Input: dimensioned drawing with shaded views. Units: mm. Origin: part minimum x, y, z. A direction names the side the tool comes from. Round coordinates to 2 decimals unless told otherwise and drop trailing zeros. Loops run counter-clockwise (first coordinate to the right, second up) from the corner with the lowest first, then second, coordinate; pieces in that order, holes last.
Item 1: Ray query, L1, parallel to X at y = 1.5, z = 6; L2, parallel to X at y = 0.8, z = 11; L3, parallel to X at y = 0.25, z = 13.25. Return the intervals inside material, ascending.
Item 2: First-contact query: P1, Ø0.8, axis at y = 0.5, z = 7, coming from the +X side; P2, Ø1.1, axis at y = 0.5, z = 8.5, coming from the -X side. Flat tips, straight axial feed; report the tip coordinate or a pass-through.
Item 3: Section query B-B on z = 10.5. Return loops of the section in (x, y), then the cut area to 3 significant figures.
Item 4: Pull-direction query (X, two-part tool) for the marked faces 1 and 2; classes: released by +X, released by -X, zero draft, split by the parting line, or undercut.
Item 5: Section query A-A on y = 0.6. Return loops of the section in (x, z).
Item 6: Section query C-C on x = 23.5. Return loops of the section in (y, z).
Item 7: Section query D-D on z = 12.25. Return loops of the section in (x, y), then the cut area to 3 significant figures.
Item 8: Access query for the marked faces 3 and 4. Directions: +Z, -Z, +X, -X, +Y, -Y. A direction counts if a zero-diameter tool reaches every point of the face in a straight line with its end or side. Return the directions, or none.
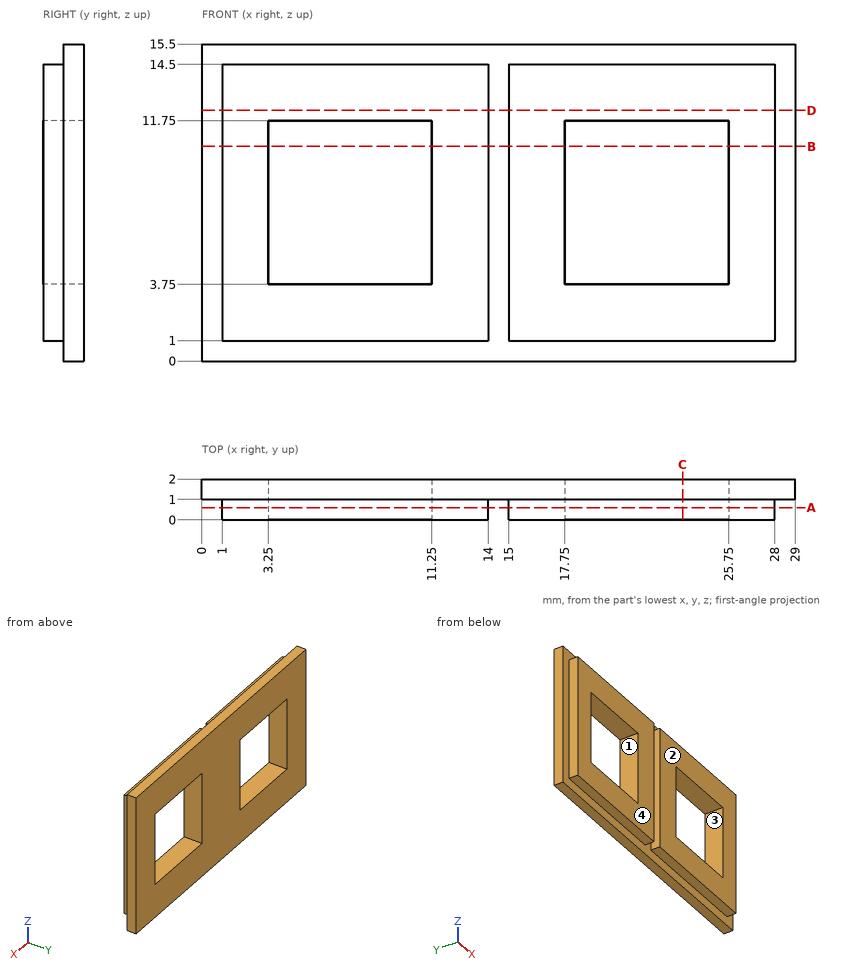
Data:
1. L1: x = 0 to 3.25, 11.25 to 17.75, 25.75 to 29
1. L2: x = 1 to 3.25, 11.25 to 14, 15 to 17.75, 25.75 to 28
1. L3: x = 1 to 14, 15 to 28
2. P1: stops at x = 28
2. P2: stops at x = 0
3. outline: (0, 1) - (1, 1) - (1, 0) - (3.25, 0) - (3.25, 2) - (0, 2) - close; (11.25, 0) - (14, 0) - (14, 1) - (15, 1) - (15, 0) - (17.75, 0) - (17.75, 2) - (11.25, 2) - close; (25.75, 0) - (28, 0) - (28, 1) - (29, 1) - (29, 2) - (25.75, 2) - close
3. area: 23.0 mm2
4. face 1: undercut
4. face 2: zero draft
5. outline: (1, 1) - (14, 1) - (14, 14.5) - (1, 14.5) - close; (15, 1) - (28, 1) - (28, 14.5) - (15, 14.5) - close; hole (3.25, 3.75) - (11.25, 3.75) - (11.25, 11.75) - (3.25, 11.75) - close; hole (17.75, 3.75) - (25.75, 3.75) - (25.75, 11.75) - (17.75, 11.75) - close
6. outline: (0, 1) - (1, 1) - (1, 0) - (2, 0) - (2, 3.75) - (0, 3.75) - close; (0, 11.75) - (2, 11.75) - (2, 15.5) - (1, 15.5) - (1, 14.5) - (0, 14.5) - close
7. outline: (0, 1) - (1, 1) - (1, 0) - (14, 0) - (14, 1) - (15, 1) - (15, 0) - (28, 0) - (28, 1) - (29, 1) - (29, 2) - (0, 2) - close
7. area: 55.0 mm2
8. face 3: +Y, -Y
8. face 4: +Z, -Z, +X, -X, -Y
